Geometry check sheet. Reference: drawing and pictorial views, mm from the part's lowest x, y, z. Give positions to 0.01 mm unless a question says otherwise; leave off trailing zeros. Order: outer loops, then holes, each group sorted by start corner. A loop starts at its lowest first (then second) coordinate and runs counter-clockwise, first axis right, second up.
Item 1: Sectioned sample at A-A on x = 63.6. Record the boundary of the cut face in (y, z).
Item 2: Material ranges on line 1 along X through (y, z) = (1.45, 9.75); line 2 along X through (y, z) = (1.1, 8); line 3 along X through (y, z) = (0.55, 2.6), recorded low to high.
Item 3: Sectioned sample at D-D on x = 41.5. Record the boundary of the cut face in (y, z).
Item 4: Gauge pin test, flat ends, axial feed: P1, Ø2, axis at x = 63.6, z = 9.6, coming from the -Y side; P2, Ø0.6, axis at x = 40.5, y = 1.5, coming from the +Z side. Record the tip position at first contact, or that the pin passes through.
Item 5: Sectioned sample at B-B on y = 0.35. Record the boundary of the cut face in (x, z).
Item 6: Sectioned sample at C-C on z = 2.6. Record the boundary of the cut face in (x, y), and give its area (3 significant figures).
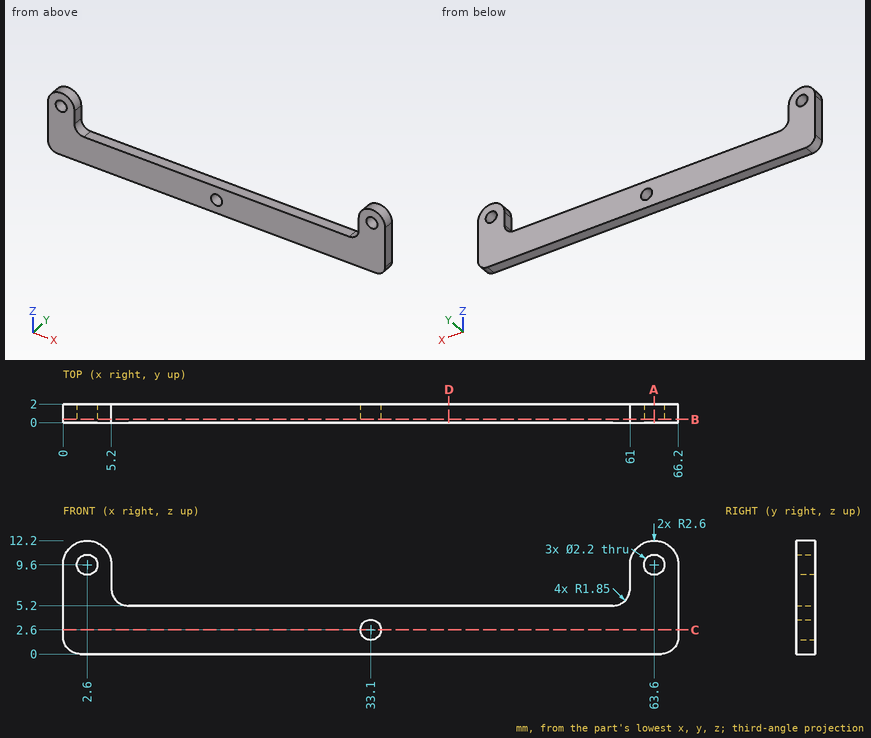
Report:
1. outline: (0, 0) - (2, 0) - (2, 8.5) - (0, 8.5) - close; (0, 10.7) - (2, 10.7) - (2, 12.2) - (0, 12.2) - close
2. line 1: x = 0 to 1.51, 3.69 to 5.2, 61 to 62.51, 64.69 to 66.2
2. line 2: x = 0 to 5.2, 61 to 66.2
2. line 3: x = 0 to 32, 34.2 to 66.2
3. outline: (0, 0) - (2, 0) - (2, 5.2) - (0, 5.2) - close
4. P1: passes through
4. P2: stops at z = 5.2
5. outline: (0, 1.85) arc R1.85 ccw to (1.85, 0) - (64.35, 0) arc R1.85 ccw to (66.2, 1.85) - (66.2, 9.6) arc R2.6 ccw to (61, 9.6) - (61, 7.05) arc R1.85 cw to (59.15, 5.2) - (7.05, 5.2) arc R1.85 cw to (5.2, 7.05) - (5.2, 9.6) arc R2.6 ccw to (0, 9.6) - close; hole circle Ø2.2 at (2.6, 9.6); hole circle Ø2.2 at (33.1, 2.6); hole circle Ø2.2 at (63.6, 9.6)
6. outline: (0, 0) - (32, 0) - (32, 2) - (0, 2) - close; (34.2, 0) - (66.2, 0) - (66.2, 2) - (34.2, 2) - close
6. area: 128 mm2
